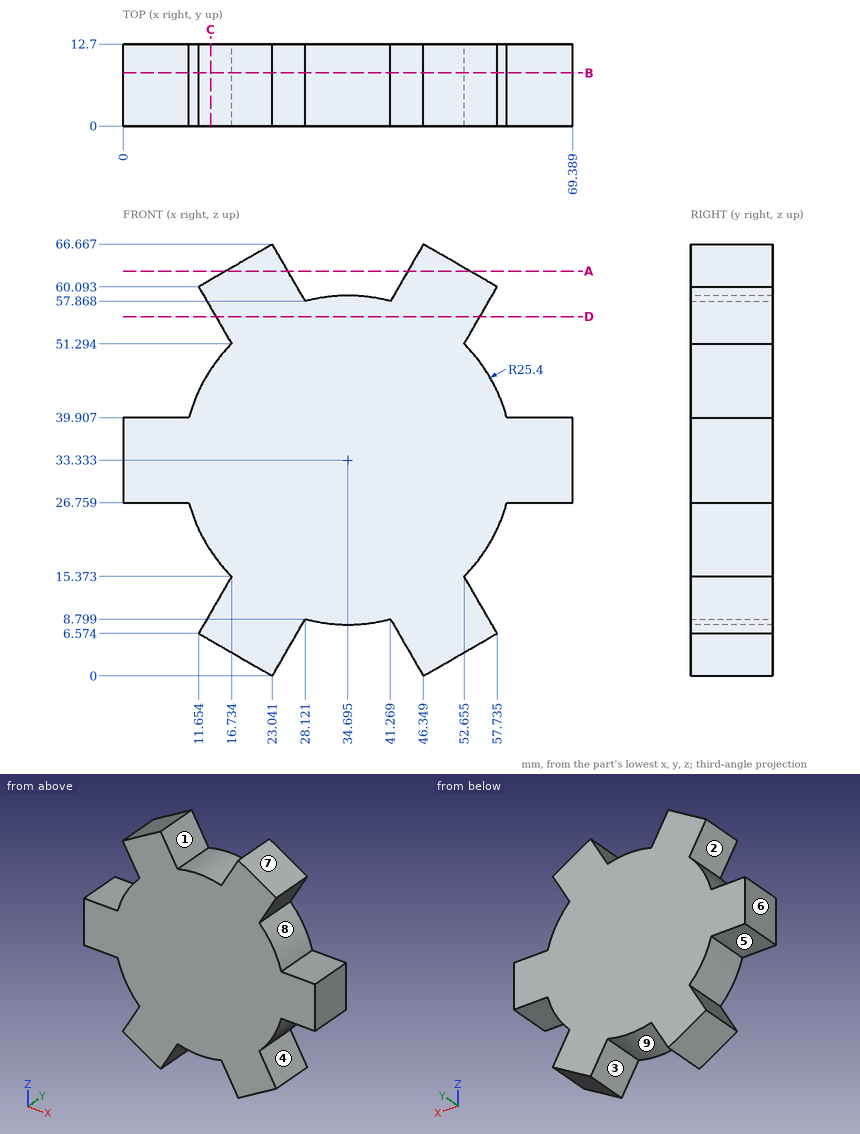
Here's the drawing with two shaded views (mm, measured from the low corner). I have some questions. A direction names the side the tool comes from. Round coordinates to 2 decimals unless told otherwise and drop trailing zeros. Loops run counter-clockwise (first coordinate to the right, second up) from the corner with the lowest first, then second, coordinate; pieces in that order, holes last. Notation, with made-up numbers: M 87,-16 L 124,-16 A20 cw 124,0 Z; hole C -18.5,6 d4. An arc over 180 degrees is marked long. Answer as a JSON object with one key per item and string values. Group by question number.
Q1. Imagine slicing it at C-C, the plane x = 13.5. Please give me the cut outline in (y, z) (1 decimal).
Q2. We'd pull the mould along Z, two halves only. Please class the marked faces 6, 7, 8 and 9: +Z half, -Z half, draft (parallel to the pull), parting line (faces both ways), or undercut.
Q3. Will these pins go through, and if not, where does the flat tip stop? pin 1 (1 mm diameter, centred on x = 43, y = 10, fed in from +Z) (1 decimal); pin 2 (5 mm diameter, centred on y = 10, z = 14.5, fed in from +X); pin 3 (5 mm diameter, centred on x = 66.5, y = 7, fed in from +Z).
Q4. Imagine slicing it at B-B, the plane y = 8.25. Please give me the cut outline in (x, z) (1 decimal).
Q5. On a 3-axis mill with a long thin cutter (end or side, diameter ignored), from which of +Z, -Z, +X, -X, +Y, -Y can I reach the whole of each face in a straight line? I mean the marked faces 1, 2, 3, 4 and 5. Say none if no direction works.
Q6. Imagine slicing it at A-A, the plane z = 62.5. Please give me the cut outline in (x, y) (1 decimal), then the cut area to 3 significant figures.
Q7. Please list where these lines run through material, in increasing order: L1, parallel to Z at x = 53, y = 9.5 (1 decimal); L2, parallel to Z at x = 9, y = 9; L3, parallel to X at y = 2.5, z = 6.5 (1 decimal).
Q8. Imagine slicing it at D-D, the plane z = 55.5. Please give me the cut outline in (x, y) (1 decimal), then the cut area to 3 significant figures.
Findings:
{
 "1": {"outline": "M 0,5.5 L 12.7,5.5 L 12.7,9.8 L 0,9.8 Z; M 0,19.3 L 12.7,19.3 L 12.7,47.3 L 0,47.3 Z; M 0,56.9 L 12.7,56.9 L 12.7,61.2 L 0,61.2 Z"},
 "2": {"face 6": "draft", "face 7": "+Z half", "face 8": "undercut", "face 9": "-Z half"},
 "3": {"pin 1": "stops at z = 61.7", "pin 2": "stops at x = 54.6", "pin 3": "stops at z = 39.91"},
 "4": {"outline": "M 0,26.8 L 10.2,26.8 A25.4 ccw 16.7,15.4 L 11.7,6.6 L 23,0 L 28.1,8.8 A25.4 ccw 41.3,8.8 L 46.3,0 L 57.7,6.6 L 52.7,15.4 A25.4 ccw 59.2,26.8 L 69.4,26.8 L 69.4,39.9 L 59.2,39.9 A25.4 ccw 52.7,51.3 L 57.7,60.1 L 46.3,66.7 L 41.3,57.9 A25.4 ccw 28.1,57.9 L 23,66.7 L 11.7,60.1 L 16.7,51.3 A25.4 ccw 10.2,39.9 L 0,39.9 Z"},
 "5": {"face 1": "+Z, +Y, -Y", "face 2": "-X, +Y, -Y", "face 3": "-Z, +Y, -Y", "face 4": "+X, +Y, -Y", "face 5": "-Z, -X, +Y, -Y"},
 "6": {"outline": "M 15.8,0 L 25.4,0 L 25.4,12.7 L 15.8,12.7 Z; M 43.9,0 L 53.6,0 L 53.6,12.7 L 43.9,12.7 Z", "area": "244 mm2"},
 "7": {"L1": "z = 3.8 to 14.8, 15.7 to 50.9, 51.9 to 62.8", "L2": "z = 26.76 to 39.91", "L3": "x = 11.8 to 26.8, 42.6 to 57.6"},
 "8": {"outline": "M 14.3,0 L 55.1,0 L 55.1,12.7 L 14.3,12.7 Z", "area": "518 mm2"}
}
